Part model, mm, in its own coordinate system. A direction names the side the tool comes from. Give positions to 0.01 mm unless a question says otherwise; leave off trailing zeros. Order: outer loops, then holes, each group sorted by start corner. A loop starts at its lowest first (then second) coordinate and runs counter-clockwise, first axis right, second up. Notation, with made-up numbers: (62, 65) - (74, 65) arc R12 ccw to (74, 84) - close; hole circle Ø4 at (24.5, 8.25). An arc over 180 degrees is marked (long way). Use one line per item in the form item = value. Start each with the question number.
1. Band-saw the part on C-C, the plane z = 0. List the corners of the cut face in (x, y).
2. Band-saw the part on A-A, the plane y = 45. List the corners of the cut face in (x, z), plus the area to 3 significant figures.
3. Band-saw the part on B-B, the plane y = 90. List the corners of the cut face in (x, z), plus the area to 3 significant figures.
4. Pull direction X, two halves, no side cores. Call faces 6 (the face through (-4.197, 49, -18)), 7 (the face through (11, 123, -4)), 8 (the face through (-7, 54.501, -17)): +X half, -X half, draft (parallel to the pull), parting line (faces both ways), or undercut.
5. Drill centre lines: line 1 (Y direction, x = -18, z = 0); line 2 (Y direction, x = 1.5, z = 15.5); line 3 (X direction, y = 75.5, z = 0.5). Where is each one in solid material? Low to high.
6. Band-saw the part on D-D, the plane z = 8. List the corners of the cut face in (x, y), plus the area to 3 significant figures.
7. Tool access for faces 1 (the face through (-17.05, 69.3, 3.86)), 2 (the face through (-7, 43.786, -17)), 3 (the face through (3, 88.732, 18)), 4 (the face through (0, 122, -16.9)), 5 (the face through (0, 122, -12)): list every direction of +Z, -Z, +X, -X, +Y, -Y with a clear straight run to the whole face (end or side of a thin tool).
8. Pin check, flat tips, straight feed: P1, Ø10, axis at x = 5.5, z = -5, coming from the -Y side; P2, Ø2.5, axis at x = 0.5, y = 121, coming from the -Z side; P3, Ø3.5, axis at y = 121, z = -15.5, coming from the +X side; P4, Ø1.7, axis at y = 48, z = -18, coming from the -X side. Stop position of each tip, or through.
from build123d import *
from build123d.topology import SkipClean

# Parameters (mm, degrees)
BOSS_EXTRUDE1_DEPTH = 120
SKETCH13_R          = 19.5
SKETCH13_R_2        = 10.25
BOSS_EXTRUDE3_DEPTH = 3
SKETCH16_W          = 6.1
SKETCH16_H          = 4.9
CUT_EXTRUDE1_DEPTH  = 5
SKETCH17_W          = 8
SKETCH17_H          = 15
CUT_EXTRUDE2_DEPTH  = 150
SKETCH18_R          = 6
CUT_EXTRUDE5_DEPTH  = 20
SKETCH21_W          = 5.844351091
SKETCH21_H          = 10.714643668
CUT_EXTRUDE6_DEPTH  = 120
BOSS_EXTRUDE4_DEPTH = 10


with BuildPart() as part:
    # Sketch12 → Boss-Extrude1 (new body)
    with BuildSketch(Plane(origin=(0, 0, 0), x_dir=(1, 0, 0), z_dir=(0, 1, 0))):
        with BuildLine():
            Line((8.634693417, 15.51841097), (8.20840412, 17.688191027))
            ThreePointArc((8.20840412, 17.688191027), (-19.139762737, -3.730882249), (14.250877044, -13.310240549))
            Line((14.250877044, -13.310240549), (13.836638735, -11.183931196))
            Line((13.836638735, -11.183931196), (12.790172439, -11.44177067))
            Line((12.790172439, -11.44177067), (12.971781009, -12.381940525))
            Line((12.971781009, -12.381940525), (12.217996211, -12.500838715))
            ThreePointArc((12.217996211, -12.500838715), (-17.156357674, -3.348102652), (6.621374847, 16.1773853))
            Line((6.621374847, 16.1773853), (7.375159644, 16.345842711))
            Line((7.375159644, 16.345842711), (7.567993782, 15.364331637))
            Line((7.567993782, 15.364331637), (8.634693417, 15.51841097))
        make_face()
    extrude(amount=BOSS_EXTRUDE1_DEPTH)

    # Sketch13 → Boss-Extrude3 (add)
    with BuildSketch(Plane(origin=(0, 120, 0), x_dir=(1, 0, 0), z_dir=(0, 1, 0))):
        with Locations(Location((0, 0, 0), (0, 0, 65.10581206))):
            Circle(SKETCH13_R)
        with Locations(Location((0, 0, 0), (0, 0, 270))):
            Circle(SKETCH13_R_2, mode=Mode.SUBTRACT)
    extrude(amount=BOSS_EXTRUDE3_DEPTH)

    # Sketch16 → Cut-Extrude1 (cut)
    with BuildSketch(Plane(origin=(0, 123, 0), x_dir=(1, 0, 0), z_dir=(0, 1, 0))):
        with Locations((0, 14.45)):
            Rectangle(SKETCH16_W, SKETCH16_H)
    extrude(amount=-CUT_EXTRUDE1_DEPTH, mode=Mode.SUBTRACT)

    # Sketch17 → Cut-Extrude2 (cut)
    with BuildSketch(Plane.XY):
        with Locations((3.376565864, 81.232231727)):
            Rectangle(SKETCH17_W, SKETCH17_H)
    extrude(amount=CUT_EXTRUDE2_DEPTH, mode=Mode.SUBTRACT)

    # Sketch18 → Cut-Extrude5 (cut)
    with BuildSketch(Plane(origin=(0, 0, 0), x_dir=(0, 0, -1), z_dir=(1, 0, 0))):
        with Locations((0, 110.771126565)):
            Circle(SKETCH18_R)
    extrude(amount=-CUT_EXTRUDE5_DEPTH, mode=Mode.SUBTRACT)

    # Sketch21 → Cut-Extrude6 (cut)
    with BuildSketch(Plane.XY):
        with Locations((-7.11941315, 49.143528952)):
            Rectangle(SKETCH21_W, SKETCH21_H)
    extrude(amount=-CUT_EXTRUDE6_DEPTH, mode=Mode.SUBTRACT)

    # Sketch24 → Boss-Extrude4 (add)
    with SkipClean():  # the faces are left unmerged after this step: merging them gives an invalid solid
        with BuildSketch(Plane(origin=(0, 10, 0), x_dir=(-1, 0, 0), z_dir=(0, -1, 0))):
            with BuildLine():
                Line((-8.634693417, 15.51841097), (-7.567993782, 15.364331637))
                Line((-7.567993782, 15.364331637), (-7.375159644, 16.345842711))
                Line((-7.375159644, 16.345842711), (-6.711023244, 15.718008714))
                ThreePointArc((-6.711023244, 15.718008714), (16.685830266, -3.494713985), (-12.217996211, -12.500838715))
                Line((-12.217996211, -12.500838715), (-12.971781009, -12.381940525))
                Line((-12.971781009, -12.381940525), (-12.790172439, -11.44177067))
                Line((-12.790172439, -11.44177067), (-13.836638735, -11.183931196))
                Line((-13.836638735, -11.183931196), (-14.250877044, -13.310240549))
                ThreePointArc((-14.250877044, -13.310240549), (19.139762737, -3.730882249), (-8.20840412, 17.688191027))
                Line((-8.20840412, 17.688191027), (-8.634693417, 15.51841097))
            make_face()
        extrude(amount=-BOSS_EXTRUDE4_DEPTH)


solid = part.part
From the geometry:
q1.outline = (-19.5, 0) - (-17.48, 0) - (-17.48, 10) - (-17, 10) - (-17, 20) - (-17.48, 20) - (-17.48, 104.77) - (-19.5, 104.77) - close; (-19.5, 116.77) - (-17.48, 116.77) - (-17.48, 120) - (-10.25, 120) - (-10.25, 123) - (-19.5, 123) - close; (10.25, 120) - (19.5, 120) - (19.5, 123) - (10.25, 123) - close
q2.outline = (-10.04, -16.72) - (-10.04, -14.31) arc R17.48 cw (long way) to (12.22, 12.5) - (12.97, 12.38) - (12.79, 11.44) - (13.84, 11.18) - (14.25, 13.31) arc R19.5 ccw (long way) to start; (-4.2, -19.04) arc R19.5 ccw to (8.21, -17.69) - (8.63, -15.52) - (7.57, -15.36) - (7.38, -16.35) - (6.62, -16.18) arc R17.48 cw to (-4.2, -16.97) - close
q2.area = 154 mm²
q3.outline = (6.62, -16.18) arc R17.48 cw (long way) to (12.22, 12.5) - (12.97, 12.38) - (12.79, 11.44) - (13.84, 11.18) - (14.25, 13.31) arc R19.5 ccw (long way) to (8.21, -17.69) - (8.63, -15.52) - (7.57, -15.36) - (7.38, -16.35) - close
q3.area = 167 mm²
q4.face_6 = -X half
q4.face_7 = draft
q4.face_8 = undercut
q5.line_1 = 0 to 104.77, 116.77 to 123
q5.line_2 = 120 to 123
q5.line_3 = -19.49 to -17.47
q6.outline = (-17.78, 0) - (-15.54, 0) - (-15.54, 10) - (-15.13, 10) - (-15.13, 20) - (-15.54, 20) - (-15.54, 120) - (-6.41, 120) - (-6.41, 123) - (-17.78, 123) - close; (6.41, 120) - (17.78, 120) - (17.78, 123) - (6.41, 123) - close
q6.area = 341 mm²
q7.face_1 = none
q7.face_2 = -Z
q7.face_3 = +Z
q7.face_4 = +Y
q7.face_5 = +Y, -Y
q8.P1 = 120
q8.P2 = -19.5
q8.P3 = 13.83
q8.P4 = -4.2
